CAD build for the part. Positions are in the model's coordinates, mm. A direction names the side the tool comes from. Round coordinates to 2 decimals unless told otherwise and drop trailing zeros. Order: outer loops, then holes, each group sorted by start corner. A loop starts at its lowest first (then second) coordinate and runs counter-clockwise, first axis right, second up. Notation, with made-up numbers: M 21.5,-25.5 L 76.5,-25.5 A22 cw 76.5,1.5 Z; hole C -17.75,74.25 d11. An arc over 180 degrees is marked long. Answer as a JSON object with one key per item and string values. Group by question number.
```python
from build123d import *

# Parameters (mm, degrees)
F2_R = 3.868


with BuildPart() as f3:
    # F3: sweep along a path in F0
    with BuildLine(Plane.XY) as f3_path:
        Line((0, 0), (25, 0))
        ThreePointArc((25, 0), (28.5355339059, -1.4644660941), (30, -5))
        Line((30, -5), (30, -46.2890183416))
        ThreePointArc((30, -46.2890183416), (29.0149889262, -49.2689283944), (26.448054431, -51.0747406868))
        Line((26.448054431, -51.0747406868), (-119.5911694754, -95.2630011068))
        ThreePointArc((-119.5911694754, -95.2630011068), (-122.1581039705, -97.0688133992), (-123.1431150443, -100.0487234519))
        Line((-123.1431150443, -100.0487234519), (-123.1431150443, -166.3377417936))
    # F2 (on line) → F3 (sweep)
    with BuildSketch(Plane.XZ.offset(166.3377417936)):
        with Locations((-122.8476336243, 0)):
            Circle(F2_R)
    sweep(path=f3_path.line)


solid = f3.part
```
Item 1: Cut at A-A, the plane z = 0. Give the cut face in (x, y).
Item 2: Flat gauge pins, fed straight in: pin 1 Ø3 at (y, z) = (-17.5, -2.5) entering from +X; pin 2 Ø2 at (x, z) = (-35, -2) entering from -Y; pin 3 Ø4 at (y, z) = (-1.5, 0) entering from -X. Where does each tip first touch, or does it go through?
Item 3: Cut at B-B, the plane y = -32. Give the cut face in (x, z), and give its area (3 significant figures).
Item 4: Drill centre lines: line 1 (X direction, y = -13, z = 0); line 2 (X direction, y = -136.5, z = -0.5); line 3 (Y direction, x = -52, z = 2). Where is each one in solid material? Low to high. Write a range as [from, to].
Item 5: 3-axis set-ups, long thin cutter, end or side, ignore diameter. For faces 5 (the face through (0, 0, 0)), 6 (the face through (-46.44, -77.292, 1.162)): which of +Z, -Z, +X, -X, +Y, -Y reach the whole face in a straight line?
Item 6: Two-plate mould, pull along Y, no slides. Class faces 1 (the face through (-119.275, -133.657, -1.481)), 2 (the face through (26.43, -25.93, 0.17)), 3 (the face through (12.675, -0.543, -3.776)), 4 (the face through (-123, -166.338, 0)): +Y half, -Y half, draft (parallel to the pull), parting line (faces both ways), or undercut.
Response values:
{
 "1": {"outline": "M -126.72,-166.34 L -118.98,-166.34 L -118.98,-100.05 A0.84 cw -118.39,-99.25 L 27.65,-55.06 A9.16 ccw 34.16,-46.29 L 34.16,-5 A9.16 ccw 25,4.16 L 0,4.16 L 0,-3.57 L 25,-3.57 A1.43 cw 26.43,-5 L 26.43,-46.29 A1.43 cw 25.41,-47.66 L -120.63,-91.84 A8.57 ccw -126.72,-100.05 Z"},
 "2": {"pin 1": "x = 34.03", "pin 2": "y = -74", "pin 3": "x = 0"},
 "3": {"outline": "C 30.3,0 d7.74", "area": "47.0 mm^2"},
 "4": {"line 1": "[26.43, 34.16]", "line 2": "[-126.68, -119.01]", "line 3": "[-78.58, -71.66]"},
 "5": {"face 5": "+Z, -Z, -X, +Y", "face 6": "none"},
 "6": {"face 1": "draft", "face 2": "undercut", "face 3": "undercut", "face 4": "-Y half"}
}
